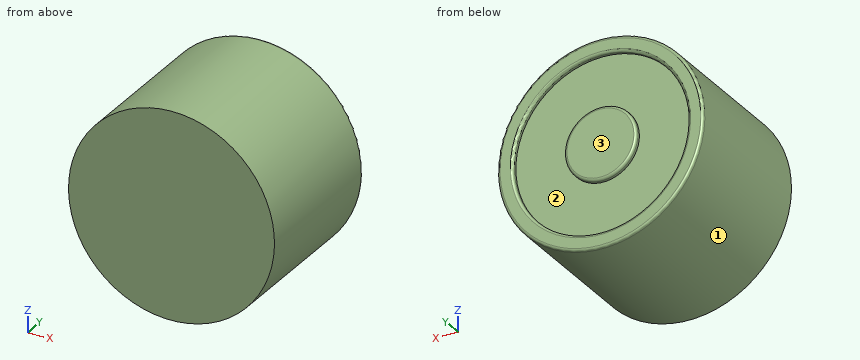
```python
from build123d import *

# Parameters (mm, degrees)
SKETCH1_R           = 10
BOSS_EXTRUDE1_DEPTH = 15
SKETCH2_R           = 8.5
CUT_EXTRUDE1_DEPTH  = 0.5
SKETCH3_R           = 3.5
BOSS_EXTRUDE2_DEPTH = 0.5
FILLET1_R           = 0.25


with BuildPart() as part:
    # Sketch1 → Boss-Extrude1 (new body)
    with BuildSketch(Plane(origin=(0, 0, 0), x_dir=(1, 0, 0), z_dir=(0, 1, 0))):
        with Locations(Location((0, 0, 0), (0, 0, 270))):
            Circle(SKETCH1_R)
    extrude(amount=BOSS_EXTRUDE1_DEPTH)

    # Sketch2 → Cut-Extrude1 (cut)
    with BuildSketch(Plane(origin=(0, 15, 0), x_dir=(1, 0, 0), z_dir=(0, 1, 0))):
        with Locations(Location((0, 0, 0), (0, 0, 270))):
            Circle(SKETCH2_R)
    extrude(amount=-CUT_EXTRUDE1_DEPTH, mode=Mode.SUBTRACT)

    # Sketch3 → Boss-Extrude2 (add)
    with BuildSketch(Plane(origin=(0, 14.5, 0), x_dir=(1, 0, 0), z_dir=(0, 1, 0))):
        with Locations(Location((0, 0, 0), (0, 0, 270))):
            Circle(SKETCH3_R)
    extrude(amount=BOSS_EXTRUDE2_DEPTH)

    # Fillet1
    fillet1_edges = [part.edges().sort_by_distance(p)[0] for p in [
        (0, 15, -3.5),
        (0, 15, -10),
        (0, 15, -8.5),
    ]]
    fillet(fillet1_edges, radius=FILLET1_R)


solid = part.part
```
Geometry check sheet. Reference: the model listing, model coordinates, mm. Face numbers are marked on the shaded views. Round coordinates to 2 decimals unless told otherwise and drop trailing zeros. Loops run counter-clockwise (first coordinate to the right, second up) from the corner with the lowest first, then second, coordinate; pieces in that order, holes last. Notation, with made-up numbers: (-36.75, 48) - (-5.75, 48) arc R24 ccw to (-5.75, 61) - close; hole circle Ø1 at (60, 59.5). An arc over 180 degrees is marked (long way). Write item = value, one per line. Start each with the question number.
1. Thickness scan on line 1 (X direction, y = 14.7, z = 0); line 2 (Y direction, x = -2.5, z = 5.5); line 3 (Y direction, x = -8.25, z = -5.25). Record the ranges inside material, lowest first.
2. Mould release check, pull along Z, two halves, no side actions. Record for the marked faces 1, 2 and 3: released by +Z, released by -Z, zero draft, split by the parting line, or undercut.
3. Depth check by flat-ended pin: pin 1 (6 mm diameter, centred on y = 11.5, z = 4, fed in from -X); pin 2 (3 mm diameter, centred on y = 7.5, z = 7, fed in from +X); pin 3 (1.5 mm diameter, centred on x = -2.5, y = 3.5, fed in from -Z). Enter the tip coordinate at first touch or a pass-through.
4. Section check B-B on z = 0. Enter the section's corners in (x, y), then the cut area to 3 significant figures.
5. Section check A-A on x = 0. Enter the section's corners in (y, z), then the cut area to 3 significant figures.
6. Section check C-C on y = 1. Enter the section's corners in (x, z), then the cut area to 3 significant figures.
Working result:
q1.line_1 = -10 to -8.5, -3.5 to 3.5, 8.5 to 10
q1.line_2 = 0 to 14.5
q1.line_3 = 0 to 15
q2.face_1 = split by the parting line
q2.face_2 = undercut
q2.face_3 = zero draft
q3.pin_1 = -9.95
q3.pin_2 = 8.35
q3.pin_3 = -9.85
q4.outline = (-10, 0) - (10, 0) - (10, 14.75) arc R0.25 ccw to (9.75, 15) - (8.75, 15) arc R0.25 ccw to (8.5, 14.75) - (8.5, 14.5) - (3.5, 14.5) - (3.5, 14.75) arc R0.25 ccw to (3.25, 15) - (-3.25, 15) arc R0.25 ccw to (-3.5, 14.75) - (-3.5, 14.5) - (-8.5, 14.5) - (-8.5, 14.75) arc R0.25 ccw to (-8.75, 15) - (-9.75, 15) arc R0.25 ccw to (-10, 14.75) - close
q4.area = 295 mm^2
q5.outline = (0, -10) - (14.75, -10) arc R0.25 ccw to (15, -9.75) - (15, -8.75) arc R0.25 ccw to (14.75, -8.5) - (14.5, -8.5) - (14.5, -3.5) - (14.75, -3.5) arc R0.25 ccw to (15, -3.25) - (15, 3.25) arc R0.25 ccw to (14.75, 3.5) - (14.5, 3.5) - (14.5, 8.5) - (14.75, 8.5) arc R0.25 ccw to (15, 8.75) - (15, 9.75) arc R0.25 ccw to (14.75, 10) - (0, 10) - close
q5.area = 295 mm^2
q6.outline = circle Ø20 at (0, 0)
q6.area = 314 mm^2
